```python
from build123d import *

# Parameters (mm, degrees)
BOSS_EXTRUDE1_DEPTH = 6
SKETCH2_R           = 422.5
CUT_EXTRUDE1_DEPTH  = 6
SKETCH3_R           = 4.5
CUT_EXTRUDE2_DEPTH  = 6
CIRPATTERN1_COUNT   = 16
SKETCH4_R           = 3
CUT_EXTRUDE3_DEPTH  = 10
SKETCH5_R           = 7.5
CUT_EXTRUDE4_DEPTH  = 10
FILLET1_R           = 6
SKETCH6_R           = 6
SKETCH6_R_2         = 4
EXTRUDE_THIN1_DEPTH = 10


with BuildPart() as part:
    # Sketch1 → Boss-Extrude1 (new body)
    with BuildSketch(Plane(origin=(0, 0, 0), x_dir=(1, 0, 0), z_dir=(0, 1, 0))):
        Polygon((315.066450454, 496.5), (497.5, 314.066450454), (497.5, -315.066450454), (315.066450454, -497.5), (-314.066450454, -497.5), (-496.5, -315.066450454), (-496.5, 314.066450454), (-314.066450454, 496.5), align=None)
    extrude(amount=BOSS_EXTRUDE1_DEPTH)

    # Sketch2 → Cut-Extrude1 (cut)
    with BuildSketch(Plane(origin=(0, 6, 0), x_dir=(1, 0, 0), z_dir=(0, 1, 0))):
        with Locations(Location((0, 0, 0), (0, 0, 270))):
            Circle(SKETCH2_R)
    extrude(amount=-CUT_EXTRUDE1_DEPTH, mode=Mode.SUBTRACT)

    # Sketch3 → Cut-Extrude2 (cut)
    with BuildSketch(Plane(origin=(0, 6, 0), x_dir=(1, 0, 0), z_dir=(0, 1, 0))):
        with Locations(Location((0, 442.5, 0), (0, 0, 270))):
            Circle(SKETCH3_R)
    cut_extrude2 = extrude(amount=-CUT_EXTRUDE2_DEPTH, mode=Mode.SUBTRACT)

    # CirPattern1: Cut-Extrude2 ×16 about axis
    cirpattern1_axis = Axis((0, 0, 0), (0, 1, 0))
    for i in range(1, CIRPATTERN1_COUNT):
        add(cut_extrude2.rotate(cirpattern1_axis, i * 360 / CIRPATTERN1_COUNT), mode=Mode.SUBTRACT)

    # Sketch4 → Cut-Extrude3 (cut)
    with BuildSketch(Plane(origin=(0, 6, 0), x_dir=(1, 0, 0), z_dir=(0, 1, 0))):
        with Locations(Location((445.5, 262.066450454, 0), (0, 0, 270))):
            Circle(SKETCH4_R)
    extrude(amount=-CUT_EXTRUDE3_DEPTH, mode=Mode.SUBTRACT)

    # Sketch5 → Cut-Extrude4 (cut)
    with BuildSketch(Plane(origin=(0, 6, 0), x_dir=(1, 0, 0), z_dir=(0, 1, 0))):
        with Locations(Location((-461.5, 244.066450454, 0), (0, 0, 270))):
            Circle(SKETCH5_R)
        with Locations(Location((462.5, -245.066450454, 0), (0, 0, 270))):
            Circle(SKETCH5_R)
    extrude(amount=-CUT_EXTRUDE4_DEPTH, mode=Mode.SUBTRACT)

    # Fillet1
    fillet1_edges = [part.edges().sort_by_distance(p)[0] for p in [
        (315.066450454, 3, -496.5),
        (497.5, 3, -314.066450454),
        (497.5, 3, 315.066450454),
        (315.066450454, 3, 497.5),
        (-314.066450454, 3, 497.5),
        (-496.5, 3, 315.066450454),
        (-496.5, 3, -314.066450454),
        (-314.066450454, 3, -496.5),
    ]]
    fillet(fillet1_edges, radius=FILLET1_R)

    # Sketch6 → Extrude-Thin1 (add)
    with BuildSketch(Plane(origin=(0, 6, 0), x_dir=(1, 0, 0), z_dir=(0, 1, 0))):
        with Locations((445.5, 262.066450454)):
            Circle(SKETCH6_R)
        with Locations((445.5, 262.066450454)):
            Circle(SKETCH6_R_2, mode=Mode.SUBTRACT)
    extrude(amount=EXTRUDE_THIN1_DEPTH)


solid = part.part
```
CAD build for the part. Positions are in the model's coordinates, mm. Coordinates: 2 decimals unless noted, no trailing zeros. Loops run counter-clockwise (first coordinate to the right, second up) from the corner with the lowest first, then second, coordinate; pieces in that order, holes last. Notation, with made-up numbers: (72.5, 86.5) - (79.5, 86.5) arc R32 ccw to (79.5, 115.5) - close; hole circle Ø2 at (-40, 26). An arc over 180 degrees is marked (long way). Return JSON: item names as keys, results as strings.
1. Band-saw the part on B-B (x = -339). Give the cut face in (y, z), and give its area (3 significant figures).
Result:
{"outline": "(0, -471.57) - (6, -471.57) - (6, -252.16) - (0, -252.16) - close; (0, 252.16) - (6, 252.16) - (6, 472.57) - (0, 472.57) - close", "area": "2,640 mm2"}
2. Probe L1, parallel to Y at x = 275, z = 357.5; L2, parallel to Z at x = 445.5, y = 9.5; L3, parallel to X at y = 5.25, z = -109.5. List the from-to ranges inside material, lowest first. Write a range as from..to.
Result:
{"L1": "y = 0..6", "L2": "z = -268.07..-266.07, -258.07..-256.07", "L3": "x = -496.5..-408.06, 408.06..497.5"}
3. Band-saw the part on C-C (y = 9.5). Give the cut face in (x, z).
Result:
{"outline": "circle Ø12 at (445.5, -262.07); hole circle Ø8 at (445.5, -262.07)"}
4. Band-saw the part on A-A (z = 334). Give the cut face in (x, y), and give its area (3 significant figures).
Result:
{"outline": "(-477.57, 0) - (-258.75, 0) - (-258.75, 6) - (-477.57, 6) - close; (258.75, 0) - (478.57, 0) - (478.57, 6) - (258.75, 6) - close", "area": "2,630 mm2"}
5. Mould opens along Z. For faces 1 (the cylindrical face through (-412.453, 3.042, -91.59)), 2 (the flat face through (-406.536, 2.958, -404.031)), 3 (the flat face through (407.536, 2.958, 405.031)) say: released by +Z, released by -Z, zero draft, split by the parting line, or undercut.
Result:
{"face 1": "undercut", "face 2": "released by -Z", "face 3": "released by +Z"}
6. Drop flat-ended pins along their axis: pin 1 (14.5 mm diameter, centred on x = -312.89, z = 312.89, fed in from +Y); pin 2 (5 mm diameter, centred on x = 368.5, z = 310.5, fed in from -Y); pin 3 (1.5 mm diameter, centred on x = -323, y = 2.5, fed in from +Z). Give the stop position or say it passes through.
Result:
{"pin 1": "stops at y = 6", "pin 2": "stops at y = 0", "pin 3": "stops at z = 489.32"}
